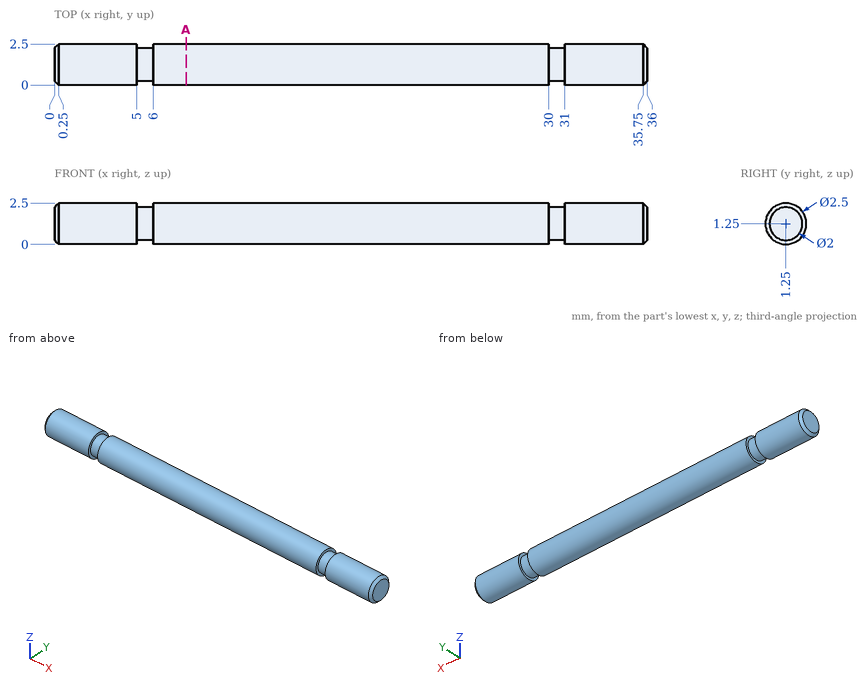
The drawing under review shows one solid part. Ordinate dimensions are in mm from its lowest x, y, z. Round coordinates to 2 decimals unless told otherwise and drop trailing zeros. Loops run counter-clockwise (first coordinate to the right, second up) from the corner with the lowest first, then second, coordinate; pieces in that order, holes last. Notation, with made-up numbers: (-14, 39.5) - (43, 39.5) arc R23 ccw to (43, 59.5) - close; hole circle Ø6 at (77, -30). An arc over 180 degrees is marked (long way). Put each result on its own line as item: value. Start each with the question number.
1. Consider section A-A on x = 8. State the section outline as (y, z) points.
2. For probe 1 along X at (y, z) = (0.3, 1.8); probe 2 along Y at (x, z) = (17.5, 1.2); probe 3 along Y at (x, z) = (33, 0.4), list the stretches that pass through material, from the lowest coordinate up. Write a range as [from, to].
3. Insertion check: P1, Ø1, axis at x = 6, z = 0.5, coming from the -Y side; P2, Ø1, axis at x = 7, z = 0.5, coming from the +Y side. Each pin has a flat end and moves straight along its axis. Give the tip position at first contact, or say it passes through.
Result sheet:
1. outline: circle Ø2.5 at (1.25, 1.25)
2. probe 1: [0.1, 5], [6, 30], [31, 35.9]
2. probe 2: [0, 2.5]
2. probe 3: [0.33, 2.17]
3. P1: y = 0.03
3. P2: y = 2.47
